Can you work these out from the model? Positions are in its coordinate system, mm. Coordinates: 2 decimals unless noted, no trailing zeros. Order: outer loops, then holes, each group sorted by start corner. A loop starts at its lowest first (then second) coordinate and runs counter-clockwise, first axis right, second up. Notation, with made-up numbers: (25.25, 19.25) -> (39.25, 19.25) arc R37 ccw to (39.25, 55.25) -> close; hole circle Ø3 at (87, 70.5). An arc over 180 degrees is marked (long way). Answer as a JSON object with one key per item and string values. Group by question number.
(1) For pin 1 (0.9 mm diameter, centred on x = 0, y = 0, fed in from -Z); pin 2 (1.5 mm diameter, centred on x = 4, z = 8.5, fed in from -Y); pin 3 (2 mm diameter, centred on y = 4.5, z = 6.5, fed in from -X); pin 4 (1 mm diameter, centred on y = -1.5, z = 3, fed in from +X), each with a flat end and sliding along its axis, tell me the tip position at first contact or that it passes through.
(2) I want a section at B-B, the plane y = -2.25. List the corners of the cut face in (x, z) for me, plus the area to 3 significant figures.
(3) I want a section at D-D, the plane y = 9. List the corners of the cut face in (x, z) for me.
(4) I want a section at A-A, the plane x = 0. List the corners of the cut face in (y, z) for me, plus the area to 3 significant figures.
(5) I want a section at C-C, the plane z = 4. List the corners of the cut face in (x, y) for me.
(6) I need wall thicknesses on line 1 (Y direction, x = 0, z = 10.75); line 2 (X direction, y = -1.25, z = 2); line 3 (Y direction, x = 3.75, z = 0.75). Which ranges of each line are inside material? Lowest first, please.
(7) If we mould it in two halves opening along X, with no side actions, what happens to faces 1 (the flat face through (-8.657, -4.994, 6.605)), 2 (the cylindrical face through (0.25, 1.48, 6.4)), 3 (the flat face through (8.65, -5, 6.6))? For each: pulls with the +X half, pulls with the -X half, needs draft (parallel to the pull), parting line crosses it, or undercut.
Autodesk Inventor part; units mm, degrees
ref_plane "YZ Plane" through (0, 0, 0) normal (1, 0, 0) x (0, 1, 0)
ref_plane "XZ Plane" through (0, 0, 0) normal (0, 1, 0) x (-1, 0, 0)
ref_plane "XY Plane" through (0, 0, 0) normal (0, 0, 1) x (1, 0, 0)
ref_plane "Work Plane1" through (8.8633, 1.5628, -1) normal (0, 0, -1) x (-1, 0, 0)
sketch "Sketch1" plane through (8.8633, 1.5628, -1) normal (0, 0, -1) x (-1, 0, 0)
  circle A0 centre (8.8633, -1.5628) radius 1.5
  circle A1 centre (8.8633, -1.5628) radius 0.55
  point P0 (8.8633, -1.5628)
extrude "Extrusion1" add sketch "Sketch1" against normal blind 15
sketch "Sketch2" plane through (0, 0, 14) normal (0, 0, 1) x (1, 0, 0)
  circle A0 centre (0, 0) radius 1.5
  line L0 (0.2764, 9.5833) -> (-0.2764, 10.4166)
  line L1 (8.1612, -5.0311) -> (9.1593, -4.969)
  line L2 (-8.4376, -4.5523) -> (-8.8829, -5.4477)
  arc A1 (8.1612, -5.0311) -> (1.5, 0.0014) centre (2.6718, -5.3723) ccw
  arc A2 (-8.4376, -4.5523) -> (-0.7487, -1.2998) centre (-5.9884, 0.3723) ccw
  arc A3 (-8.8829, -5.4477) -> (0.242, -1.4803) centre (-5.9884, 0.3723) ccw
  line L3 (-8.8829, -5.4477) -> (-8.4376, -4.5523)
  line L4 (8.1612, -5.0311) -> (9.1593, -4.969)
  circle A4 centre (3.3166, 4.9999) radius 5.4999
  circle A5 centre (3.3165, 4.9999) radius 6.4999
  circle A6 centre (2.6718, -5.3723) radius 5.5
  circle A7 centre (2.6718, -5.3725) radius 6.5001
  circle A8 centre (-5.9884, 0.3723) radius 6.5
  circle A9 centre (-5.9884, 0.3721) radius 5.4999
  arc A10 (-0.2764, 10.4166) -> (-1.403, 0.5306) centre (3.3167, 5) ccw
  arc A11 (0.2764, 9.5833) -> (-0.7512, 1.2983) centre (3.3167, 5) ccw
  arc A12 (9.1593, -4.969) -> (1.161, 0.9497) centre (2.6718, -5.3723) ccw
  point P0 (0, 0)
  point P1 (-2.459, 2.3282)
extrude "Extrusion2" add sketch "Sketch2" against normal blind 15 contours A0 A7 A4 A1 | A4 A7 A5 A1 | A5 A7 L1 A1 | A8 A5 L0 A4 | A4 A9 A5 A8 | A3 A6 A2 A0 | A0 A5 A9 A4 | A3 A7 A2 A6 | L2 A2 A7 A3
sketch "Sketch4" plane through (8.8633, 1.5628, 14) normal (0, 0, 1) x (1, 0, 0)
  point P0 (-8.8633, -1.5628)
properties part number "pump_impeller"
Computed values:
{
 "1": {"pin 1": "passes through", "pin 2": "stops at y = -0.28", "pin 3": "stops at x = -3.18", "pin 4": "stops at x = 8.23"},
 "2": {"outline": "(-1.15, -1) -> (-0.04, -1) -> (-0.04, 14) -> (-1.15, 14) -> close; (7.2, -1) -> (8.37, -1) -> (8.37, 14) -> (7.2, 14) -> close", "area": "34.3 mm2"},
 "3": {"outline": "(-1.81, -1) -> (-0.46, -1) -> (-0.46, 14) -> (-1.81, 14) -> close"},
 "4": {"outline": "(-2.16, -1) -> (-0.55, -1) -> (-0.55, 14) -> (-2.16, 14) -> close; (0.55, -1) -> (1.5, -1) -> (1.5, 14) -> (0.55, 14) -> close; (9.39, -1) -> (10, -1) -> (10, 14) -> (9.39, 14) -> close", "area": "47.5 mm2"},
 "5": {"outline": "(-8.88, -5.45) arc R6.5 ccw to (0.24, -1.48) arc R1.5 ccw to (1.5, 0) arc R5.5 cw to (8.16, -5.03) -> (9.16, -4.97) arc R6.5 ccw to (1.16, 0.95) arc R1.5 ccw to (-0.75, 1.3) arc R5.5 cw to (0.28, 9.58) -> (-0.28, 10.42) arc R6.5 ccw to (-1.4, 0.53) arc R1.5 ccw to (-0.75, -1.3) arc R5.5 cw to (-8.44, -4.55) -> close; hole circle Ø1.1 at (0, 0)"},
 "6": {"line 1": "y = -2.16 to -0.55, 0.55 to 1.5, 9.39 to 10", "line 2": "x = -0.83 to 0.83, 6.31 to 7.7", "line 3": "y = 0.02 to 1.04"},
 "7": {"face 1": "pulls with the -X half", "face 2": "undercut", "face 3": "pulls with the +X half"}
}
